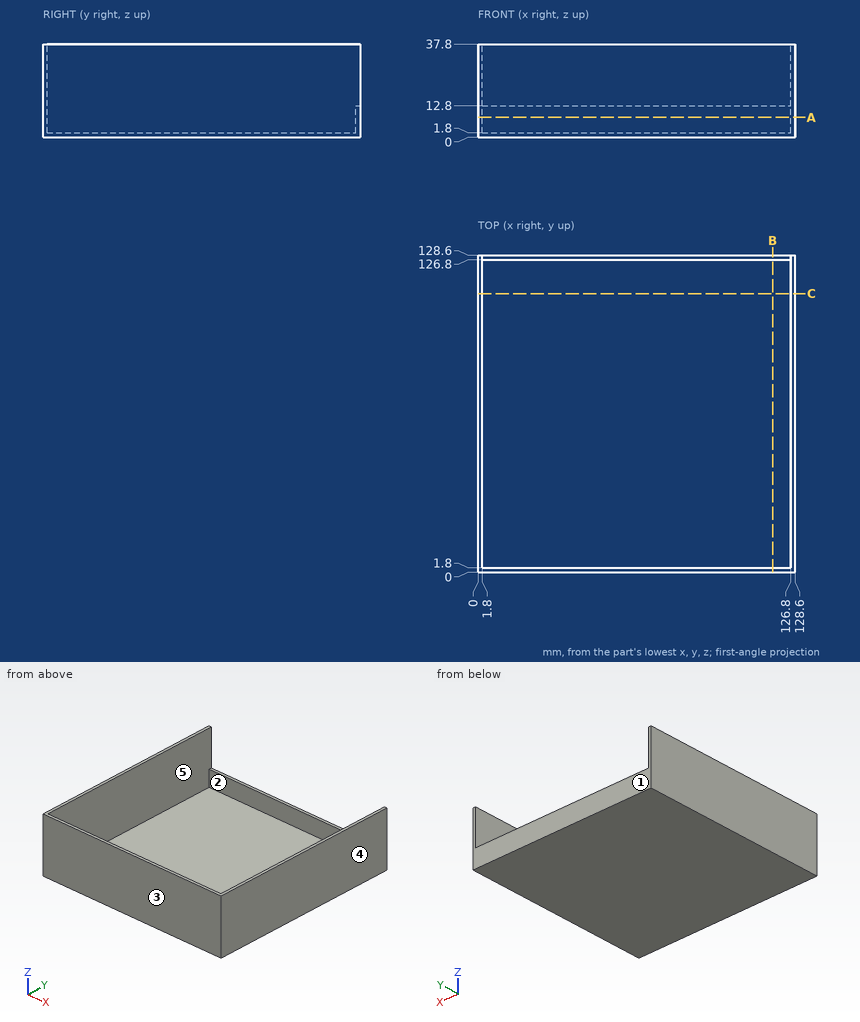
Print and shaded views of the part. All mm, measured from the part's lowest x, y and z. A direction names the side the tool comes from. Coordinates: 2 decimals unless noted, no trailing zeros. Order: outer loops, then holes, each group sorted by start corner. A loop starts at its lowest first (then second) coordinate and runs counter-clockwise, first axis right, second up. Notation, with made-up numbers: (-21.5, 73.5) -> (31.5, 73.5) arc R13 ccw to (31.5, 87.5) -> close; hole circle Ø5 at (3, 78). An arc over 180 degrees is marked (long way). Use one line per item in the form item = value. Start each with the question number.
1) Band-saw the part on A-A on z = 8. Give the cut face in (x, y).
2) Drop flat-ended pins along their axis: pin 1 (3 mm diameter, centred on y = 37, z = 6, fed in from -X); pin 2 (3 mm diameter, centred on x = 50, y = 41.5, fed in from +Z); pin 3 (1.4 mm diameter, centred on x = 42, y = 127.5, fed in from +Z). Give the stop position or say it passes through.
3) Pull direction Y, two halves, no side cores. Call the marked faces 3, 4 and 5: +Y half, -Y half, draft (parallel to the pull), parting line (faces both ways), or undercut.
4) Band-saw the part on B-B on x = 119.5. Give the cut face in (y, z).
5) Drill centre lines: L1, parallel to Y at x = 82, z = 10; L2, parallel to Y at x = 18.5, z = 33. Where is each one in solid material? Low to high. Write a range as [from, to].
6) Band-saw the part on C-C on y = 113. Give the cut face in (x, z), then the cut area to 3 significant figures.
7) Tool access for the marked faces 1 and 2: list every direction of +Z, -Z, +X, -X, +Y, -Y with a clear straight run to the whole face (end or side of a thin tool).
Entries:
q1.outline = (0, 0) -> (128.6, 0) -> (128.6, 128.6) -> (0, 128.6) -> close; hole (1.8, 1.8) -> (126.8, 1.8) -> (126.8, 126.8) -> (1.8, 126.8) -> close
q2.pin_1 = 0
q2.pin_2 = 1.8
q2.pin_3 = 12.8
q3.face_3 = -Y half
q3.face_4 = draft
q3.face_5 = undercut
q4.outline = (0, 0) -> (128.6, 0) -> (128.6, 12.8) -> (126.8, 12.8) -> (126.8, 1.8) -> (1.8, 1.8) -> (1.8, 37.8) -> (0, 37.8) -> close
q5.L1 = [0, 1.8], [126.8, 128.6]
q5.L2 = [0, 1.8]
q6.outline = (0, 0) -> (128.6, 0) -> (128.6, 37.8) -> (126.8, 37.8) -> (126.8, 1.8) -> (1.8, 1.8) -> (1.8, 37.8) -> (0, 37.8) -> close
q6.area = 361 mm2
q7.face_1 = +Z, -Z, +X, -X, +Y
q7.face_2 = +Z
